Geometry: see drawing. Coordinates: mm, zero at the bounding-box minimum. A direction names the side the tool comes from. Give positions to 0.01 mm unless a question says otherwise; leave off trailing zeros. Write each loop counter-clockwise with the first axis right and the second up, starting at its lowest first coordinate (ties: lowest second). Pieces come first, ordered by that corner, then holes. Notation, with made-up numbers: (48.25, 6.25) -> (92.25, 6.25) arc R7 cw to (92.25, 10.25) -> close; hole circle Ø9 at (-3.75, -29.5). An arc over 180 degrees is marked (long way). Use CSV: the item, a comma, the result in double quotes. Start each with the question number.
1) Section D-D (z = 2.8). Output: boundary loops of the cut face in (x, y), plus the area to 3 significant figures.
2) Section A-A (y = 7.5). Output: boundary loops of the cut face in (x, z), plus the area to 3 significant figures.
3) Set-up query: the marked faces 1 and 2. Return all of +Z, -Z, +X, -X, +Y, -Y with unobstructed straight access to the full face (end or side cutting, diameter ignored); none if empty.
4) Section C-C (z = 4.3). Output: boundary loops of the cut face in (x, y).
5) Draft query along X for the marked faces 3, 4 and 5. Return one class per face: pulls with the +X half, pulls with the -X half, needs draft (parallel to the pull), parting line crosses it, or undercut.
6) Material intervals for line 1 (Y direction, x = 7.5, z = 1.7); line 2 (X direction, y = 5.25, z = 1.8); line 3 (X direction, y = 6.75, z = 3.4), sorted ascending. Write a range as [from, to].
7) Contact query for a flat-ended pin moving along its axis: P1, Ø8, axis at x = 7.5, y = 7.5, coming from the +Z side. Output: stop coordinate, or through.
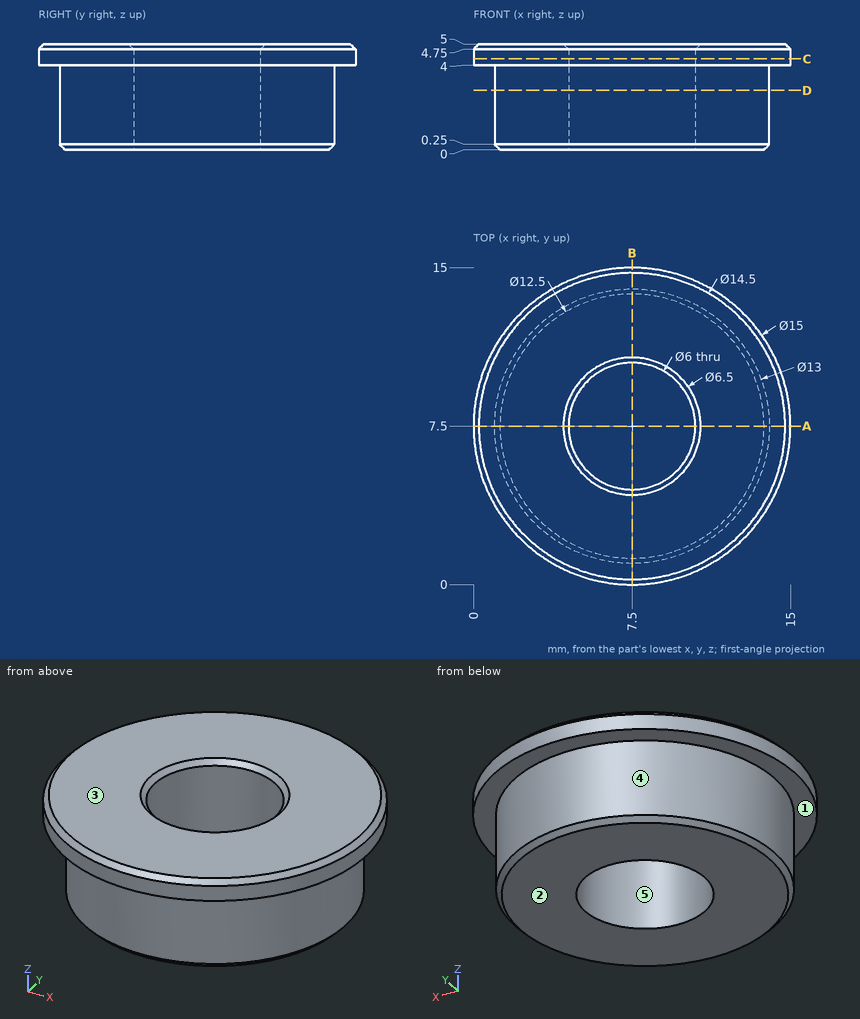
Answers follow:
1,outline,"circle Ø13 at (7.5, 7.5); hole circle Ø6 at (7.5, 7.5)"
1,area,"104 mm^2"
2,outline,"(0, 4) -> (1, 4) -> (1, 0.25) -> (1.25, 0) -> (4.5, 0) -> (4.5, 4.75) -> (4.25, 5) -> (0.25, 5) -> (0, 4.75) -> close; (10.5, 0) -> (13.75, 0) -> (14, 0.25) -> (14, 4) -> (15, 4) -> (15, 4.75) -> (14.75, 5) -> (10.75, 5) -> (10.5, 4.75) -> close"
2,area,"36.8 mm^2"
3,face 1,"-Z"
3,face 2,"-Z, +X, -X, +Y, -Y"
4,outline,"circle Ø15 at (7.5, 7.5); hole circle Ø6 at (7.5, 7.5)"
5,face 3,"needs draft"
5,face 4,"parting line crosses it"
5,face 5,"undercut"
6,line 1,"y = [1, 4.5], [10.5, 14]"
6,line 2,"x = [1.4, 5.52], [9.48, 13.6]"
6,line 3,"x = [1.04, 4.6], [10.4, 13.96]"
7,P1,"stops at z = 5"
